from build123d import *

# Parameters (mm, degrees)
CROQUIS1_R              = 2.5
SALIENTE_EXTRUIR2_DEPTH = 10
SALIENTE_EXTRUIR3_DEPTH = 10
CORTAR_EXTRUIR1_DEPTH   = 10
CROQUIS4_R              = 11.1125
CROQUIS4_R_2            = 9.525
SALIENTE_EXTRUIR4_DEPTH = 3
CROQUIS5_R              = 3
CORTAR_EXTRUIR2_DEPTH   = 10


with BuildPart() as part:
    # Croquis1 → Saliente-Extruir2 (new body)
    with BuildSketch(Plane(origin=(0, 0, 0), x_dir=(0, 0, -1), z_dir=(1, 0, 0))):
        with BuildLine():
            Line((17.5, -26), (17.5, 0))
            ThreePointArc((17.5, 0), (0, 17.5), (-17.5, 0))
            Line((-17.5, 0), (-17.5, -26))
            add(Edge.make_bspline(
                [(-17.5, -26), (0, -46), (17.5, -26)],
                knots=[0, 0, 0, 1, 1, 1], degree=2))
        make_face()
        with Locations((0, -26)):
            Circle(CROQUIS1_R, mode=Mode.SUBTRACT)
        with BuildLine():
            Line((-13.783729421, -3.874119675), (-3.536778655, 13.874119675))
            ThreePointArc((-3.536778655, 13.874119675), (-2.922822403, 14.532391234), (-2.082378285, 14.854753471))
            ThreePointArc((-2.082378285, 14.854753471), (0, 15), (2.082378285, 14.854753471))
            ThreePointArc((2.082378285, 14.854753471), (2.922822403, 14.532391234), (3.536778655, 13.874119675))
            Line((3.536778655, 13.874119675), (13.783729421, -3.874119675))
            ThreePointArc((13.783729421, -3.874119675), (14.046831188, -4.734957166), (13.905783015, -5.62398424))
            ThreePointArc((13.905783015, -5.62398424), (12.990381057, -7.5), (11.82340473, -9.230769231))
            ThreePointArc((11.82340473, -9.230769231), (11.124008785, -9.797434069), (10.246950766, -10))
            Line((10.246950766, -10), (-10.246950766, -10))
            ThreePointArc((-10.246950766, -10), (-11.124008785, -9.797434069), (-11.82340473, -9.230769231))
            ThreePointArc((-11.82340473, -9.230769231), (-12.990381057, -7.5), (-13.905783015, -5.62398424))
            ThreePointArc((-13.905783015, -5.62398424), (-14.046831188, -4.734957166), (-13.783729421, -3.874119675))
        make_face(mode=Mode.SUBTRACT)
    extrude(amount=SALIENTE_EXTRUIR2_DEPTH)

    # Croquis2 → Saliente-Extruir3 (add)
    with BuildSketch(Plane.ZY):
        with BuildLine():
            ThreePointArc((-17.5, 0), (0, -17.5), (17.5, 0))
            ThreePointArc((17.5, 0), (0, 17.5), (-17.5, 0))
        make_face()
        with BuildLine():
            Line((-13.783729421, -3.874119675), (-11.083457303, 0.802888828))
            ThreePointArc((-11.083457303, 0.802888828), (-9.6237073, 5.55625), (-6.237050773, 9.197111172))
            Line((-6.237050773, 9.197111172), (-3.536778655, 13.874119675))
            ThreePointArc((-3.536778655, 13.874119675), (-2.922822403, 14.532391234), (-2.082378285, 14.854753471))
            ThreePointArc((-2.082378285, 14.854753471), (0, 15), (2.082378285, 14.854753471))
            ThreePointArc((2.082378285, 14.854753471), (2.922822403, 14.532391234), (3.536778655, 13.874119675))
            Line((3.536778655, 13.874119675), (6.237050773, 9.197111172))
            ThreePointArc((6.237050773, 9.197111172), (9.6237073, 5.55625), (11.083457303, 0.802888828))
            Line((11.083457303, 0.802888828), (13.783729421, -3.874119675))
            ThreePointArc((13.783729421, -3.874119675), (14.046831188, -4.734957166), (13.905783015, -5.62398424))
            ThreePointArc((13.905783015, -5.62398424), (12.990381057, -7.5), (11.82340473, -9.230769231))
            ThreePointArc((11.82340473, -9.230769231), (11.124008785, -9.797434069), (10.246950766, -10))
            Line((10.246950766, -10), (4.84640653, -10))
            ThreePointArc((4.84640653, -10), (0, -11.1125), (-4.84640653, -10))
            Line((-4.84640653, -10), (-10.246950766, -10))
            ThreePointArc((-10.246950766, -10), (-11.124008785, -9.797434069), (-11.82340473, -9.230769231))
            ThreePointArc((-11.82340473, -9.230769231), (-12.990381057, -7.5), (-13.905783015, -5.62398424))
            ThreePointArc((-13.905783015, -5.62398424), (-14.046831188, -4.734957166), (-13.783729421, -3.874119675))
        make_face(mode=Mode.SUBTRACT)
        with BuildLine():
            ThreePointArc((-5.701986513, -9.538081885), (-9.290914507, -6.096438622), (-11.019569405, -1.434136107))
            ThreePointArc((-11.019569405, -1.434136107), (-11.107970902, -0.317236028), (-11.083457303, 0.802888828))
            Line((-11.083457303, 0.802888828), (-13.783729421, -3.874119675))
            ThreePointArc((-13.783729421, -3.874119675), (-14.046831188, -4.734957166), (-13.905783015, -5.62398424))
            ThreePointArc((-13.905783015, -5.62398424), (-12.990381057, -7.5), (-11.82340473, -9.230769231))
            ThreePointArc((-11.82340473, -9.230769231), (-11.124008785, -9.797434069), (-10.246950766, -10))
            Line((-10.246950766, -10), (-4.84640653, -10))
            ThreePointArc((-4.84640653, -10), (-5.279250992, -9.778402999), (-5.701986513, -9.538081885))
        make_face()
        with BuildLine():
            ThreePointArc((6.751783003, -8.82615899), (5.82871991, -9.461166971), (4.84640653, -10))
            Line((4.84640653, -10), (10.246950766, -10))
            ThreePointArc((10.246950766, -10), (11.124008785, -9.797434069), (11.82340473, -9.230769231))
            ThreePointArc((11.82340473, -9.230769231), (12.990381057, -7.5), (13.905783015, -5.62398424))
            ThreePointArc((13.905783015, -5.62398424), (14.046831188, -4.734957166), (13.783729421, -3.874119675))
            Line((13.783729421, -3.874119675), (11.083457303, 0.802888828))
            ThreePointArc((11.083457303, 0.802888828), (11.105236952, 0.401706967), (11.1125, 0))
            ThreePointArc((11.1125, 0), (11.112178614, -0.084514559), (11.111214473, -0.16902423))
            ThreePointArc((11.111214473, -0.16902423), (9.925127973, -4.997948677), (6.751783003, -8.82615899))
        make_face()
        with BuildLine():
            Line((-3.536778655, 13.874119675), (-6.237050773, 9.197111172))
            ThreePointArc((-6.237050773, 9.197111172), (-5.82871991, 9.461166971), (-5.40922796, 9.707106115))
            ThreePointArc((-5.40922796, 9.707106115), (-0.634213466, 11.094387299), (4.267786402, 10.260295097))
            ThreePointArc((4.267786402, 10.260295097), (5.279250992, 9.778402999), (6.237050773, 9.197111172))
            Line((6.237050773, 9.197111172), (3.536778655, 13.874119675))
            ThreePointArc((3.536778655, 13.874119675), (2.922822403, 14.532391234), (2.082378285, 14.854753471))
            ThreePointArc((2.082378285, 14.854753471), (0, 15), (-2.082378285, 14.854753471))
            ThreePointArc((-2.082378285, 14.854753471), (-2.922822403, 14.532391234), (-3.536778655, 13.874119675))
        make_face()
    extrude(amount=-SALIENTE_EXTRUIR3_DEPTH)

    # Croquis3 → Cortar-Extruir1 (cut)
    with BuildSketch(Plane.ZY):
        with BuildLine():
            ThreePointArc((-6.237050773, 9.197111172), (-9.6237073, 5.55625), (-11.083457303, 0.802888828))
            Line((-11.083457303, 0.802888828), (-6.237050773, 9.197111172))
        make_face()
        with BuildLine():
            ThreePointArc((11.083457303, 0.802888828), (9.6237073, 5.55625), (6.237050773, 9.197111172))
            Line((6.237050773, 9.197111172), (11.083457303, 0.802888828))
        make_face()
        with BuildLine():
            Line((4.84640653, -10), (-4.84640653, -10))
            ThreePointArc((-4.84640653, -10), (0, -11.1125), (4.84640653, -10))
        make_face()
        with BuildLine():
            ThreePointArc((-6.237050773, 9.197111172), (0, 11.1125), (6.237050773, 9.197111172))
            Line((6.237050773, 9.197111172), (11.083457303, 0.802888828))
            ThreePointArc((11.083457303, 0.802888828), (9.6237073, -5.55625), (4.84640653, -10))
            Line((4.84640653, -10), (-4.84640653, -10))
            ThreePointArc((-4.84640653, -10), (-9.6237073, -5.55625), (-11.083457303, 0.802888828))
            Line((-11.083457303, 0.802888828), (-6.237050773, 9.197111172))
        make_face()
    extrude(amount=-CORTAR_EXTRUIR1_DEPTH, mode=Mode.SUBTRACT)

    # Croquis4 → Saliente-Extruir4 (add)
    with BuildSketch(Plane.ZY):
        Circle(CROQUIS4_R)
        Circle(CROQUIS4_R_2, mode=Mode.SUBTRACT)
    extrude(amount=-SALIENTE_EXTRUIR4_DEPTH)

    # Croquis5 → Cortar-Extruir2 (cut)
    with BuildSketch(Plane(origin=(10, 0, 0), x_dir=(0, 0, -1), z_dir=(1, 0, 0))):
        with Locations((0, -26)):
            Circle(CROQUIS5_R)
    extrude(amount=-CORTAR_EXTRUIR2_DEPTH, mode=Mode.SUBTRACT)


solid = part.part
Verification items for the finished model (mm, model axes). Coordinates: 2 decimals unless noted, no trailing zeros. Order: outer loops, then holes, each group sorted by start corner. A loop starts at its lowest first (then second) coordinate and runs counter-clockwise, first axis right, second up. Notation, with made-up numbers: (7, 60.25) -> (47, 60.25) arc R32 cw to (47, 93.25) -> close; hole circle Ø4 at (-32.5, 29.5). An arc over 180 degrees is marked (long way). Put each result on its own line as item: value. Start each with the question number.
1. Mould release check, pull along Y, two halves, no side actions. Record for faces 1 (the flat face through (3, 8.3, -5)), 2 (the cylindrical face through (5.07, -28.93, 0.65)), 3 (the cylindrical face through (4.93, 17.496, -0.385)), 4 (the flat face through (5, -13, 17.5)): released by +Y, released by -Y, zero draft, split by the parting line, or undercut.
2. Cross-section at A-A, the plane y = 8. Record the boundary of the cut face in (x, z), then the cut area to 3 significant figures.
3. Cross-section at B-B, the plane z = 0. Count the separate pieces of the cut face and the enclosed holes in it, then the cut area to 3 significant figures.
4. Cross-section at D-D, the plane y = 14. Record the boundary of the cut face in (x, z), then the cut area to 3 significant figures.
5. Material ranges on L1, parallel to Y at x = 1.35, z = 0 (3 decimals); L2, parallel to Y at x = 7.25, z = 0; L3, parallel to Z at x = 7.5, y = 4.5, recorded low to high. Write a range as [from, to].
6. Go/stop test with flat-tipped pins: pin 1 Ø1 at (x, z) = (7.5, -2.5) entering from +Y; pin 2 Ø4 at (x, y) = (1, 11.5) entering from -Z; pin 3 Ø11 at (y, z) = (-4, 2) entering from +X; pin 4 Ø3.5 at (y, z) = (-26, 0) entering from +X. Record where each tip stops, or that it passes through.
Computed:
1. face 1: undercut
1. face 2: undercut
1. face 3: released by +Y
1. face 4: zero draft
2. outline: (0, -15.56) -> (10, -15.56) -> (10, -7.71) -> (3, -7.71) -> (3, -5.17) -> (0, -5.17) -> close; (0, 5.17) -> (3, 5.17) -> (3, 7.71) -> (10, 7.71) -> (10, 15.56) -> (0, 15.56) -> close
2. area: 172 mm2
3. separate pieces: 3
3. enclosed holes: 0
3. area: 262 mm2
4. outline: (0, -10.5) -> (10, -10.5) -> (10, 10.5) -> (0, 10.5) -> close
4. area: 210 mm2
5. L1: [-36, -29], [-23, -9.525], [9.525, 17.5]
5. L2: [-36, -29], [-23, -11.11], [11.11, 17.5]
5. L3: [-16.91, -10.16], [10.16, 16.91]
6. pin 1: y = 17.39
6. pin 2: z = -14.7
6. pin 3: x = 3
6. pin 4: through
